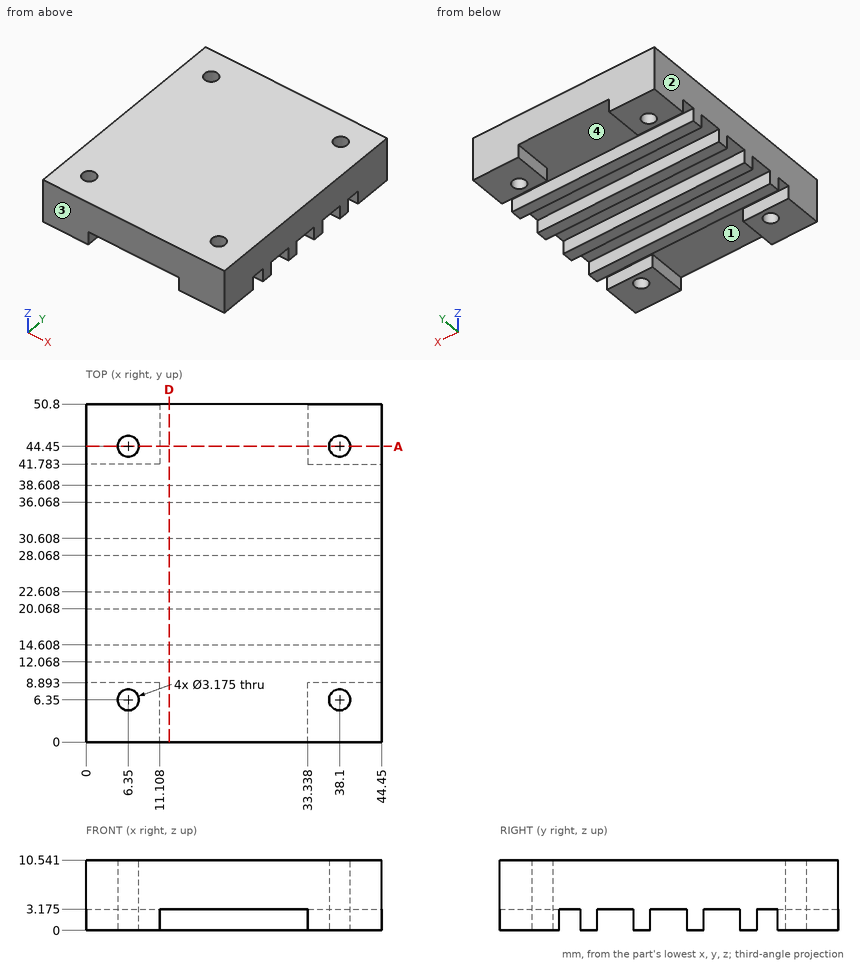
Drawing for the job (mm, zero at the part's lowest x, y, z). Give positions to 0.01 mm unless a question says otherwise; leave off trailing zeros. Loops run counter-clockwise (first coordinate to the right, second up) from the corner with the lowest first, then second, coordinate; pieces in that order, holes last. Notation, with made-up numbers: M 68.25,-36.75 L 73.25,-36.75 A10 cw 73.25,-28.75 Z; hole C -7.5,-9.75 d9. An arc over 180 degrees is marked long. Use one line per item in the form item = value.
Item 1: Drill centre lines: probe 1 along Y at (x, z) = (13.5, 1.5); probe 2 along Y at (x, z) = (6.35, 8); probe 3 along X at (y, z) = (44.45, 2.5). Where is each one in solid material? Low to high. Write a range as from..to.
Determined:
probe_1 = 12.07..14.61, 20.07..22.61, 28.07..30.61, 36.07..38.61
probe_2 = 0..4.76, 7.94..42.86, 46.04..50.8
probe_3 = 0..4.76, 7.94..11.11, 33.34..36.51, 39.69..44.45
Item 2: Slice it at A-A (y = 44.45). Count the separate pieces of the cut face and the enclosed holes in it, plus the area to 3 significant figures.
Determined:
separate_pieces = 3
enclosed_holes = 0
area = 331 mm2
Item 3: Flat gauge pins, fed straight in: pin 1 (1.9 mm diameter, centred on x = 38.1, y = 6.35, fed in from -Z); pin 2 (1 mm diameter, centred on x = 27.5, z = 1.5, fed in from +Y); pin 3 (3 mm diameter, centred on x = 15.5, y = 7, fed in from -Z) (1 decimal). Where does each tip first touch, or does it go through?
Determined:
pin_1 = through
pin_2 = 38.61
pin_3 = 3.2
Item 4: Two-plate mould, pull along Y, no slides. Class the marked faces 1, 2, 3 and 4: pulls with the +Y half, pulls with the -Y half, needs draft (parallel to the pull), parting line crosses it, or undercut.
Determined:
face_1 = undercut
face_2 = needs draft
face_3 = pulls with the -Y half
face_4 = undercut
Item 5: Slice it at D-D (x = 12.5). List the corners of the cut face in (y, z) (1 decimal).
Determined:
outline = M 0,3.2 L 12.1,3.2 L 12.1,0 L 14.6,0 L 14.6,3.2 L 20.1,3.2 L 20.1,0 L 22.6,0 L 22.6,3.2 L 28.1,3.2 L 28.1,0 L 30.6,0 L 30.6,3.2 L 36.1,3.2 L 36.1,0 L 38.6,0 L 38.6,3.2 L 50.8,3.2 L 50.8,10.5 L 0,10.5 Z
